The model under review builds one solid part; all positions refer to its coordinate system, in mm. Face numbers are marked on the shaded views. Give positions to 0.01 mm unless a question says otherwise; leave off trailing zeros. Order: outer loops, then holes, each group sorted by start corner. A loop starts at its lowest first (then second) coordinate and runs counter-clockwise, first axis right, second up. Notation, with made-up numbers: (75.5, -6.5) - (93.5, -6.5) arc R8 cw to (93.5, -0.5) - close; hole circle Ø11 at (30.25, 31.25). An arc over 180 degrees is marked (long way). Use CSV: the item, a comma, the result in double quotes.
```python
from build123d import *

# Parameters (mm, degrees)
BOSS_EXTRUDE1_DEPTH = 12.7
SKETCH2_R           = 3.175
CUT_EXTRUDE1_DEPTH  = 26.4
SKETCH3_OUTSIDE_W   = 105.562
SKETCH3_OUTSIDE_H   = 45.872
CUT_EXTRUDE4_DEPTH  = 25.4


with BuildPart() as part:
    # Sketch1 → Boss-Extrude1 (new body, symmetric)
    with BuildSketch(Plane.XY):
        with BuildLine():
            Line((-20, 0), (-42.545, 0))
            Line((-42.545, 0), (-42.545, -25.4))
            Line((-42.545, -25.4), (42.545, -25.4))
            Line((42.545, -25.4), (42.545, 0))
            Line((42.545, 0), (20, 0))
            ThreePointArc((20, 0), (0, -20), (-20, 0))
        make_face()
    extrude(amount=BOSS_EXTRUDE1_DEPTH, both=True)

    # Sketch2 → Cut-Extrude1 (cut, through all)
    with BuildSketch(Plane(origin=(0, 0, 0), x_dir=(1, 0, 0), z_dir=(0, 1, 0))):
        with Locations((-31.2725, 0)):
            Circle(SKETCH2_R)
    cut_extrude1 = extrude(amount=-CUT_EXTRUDE1_DEPTH, mode=Mode.SUBTRACT)

    # Mirror1: Cut-Extrude1 across plane
    add(cut_extrude1.mirror(Plane(origin=(0, 0, 0), x_dir=(0, 0, 1), z_dir=(1, 0, 0))), mode=Mode.SUBTRACT)

    # Sketch3 outside → Cut-Extrude4 (cut)
    with BuildSketch(Plane.XZ.offset(25.4)):
        Rectangle(SKETCH3_OUTSIDE_W, SKETCH3_OUTSIDE_H)
        with BuildLine():
            Line((-29.845, 12.7), (29.845, 12.7))
            ThreePointArc((29.845, 12.7), (42.545, 0), (29.845, -12.7))
            Line((29.845, -12.7), (-29.845, -12.7))
            ThreePointArc((-29.845, -12.7), (-42.545, 0), (-29.845, 12.7))
        make_face(mode=Mode.SUBTRACT)
    extrude(amount=-CUT_EXTRUDE4_DEPTH, mode=Mode.SUBTRACT)


solid = part.part
```
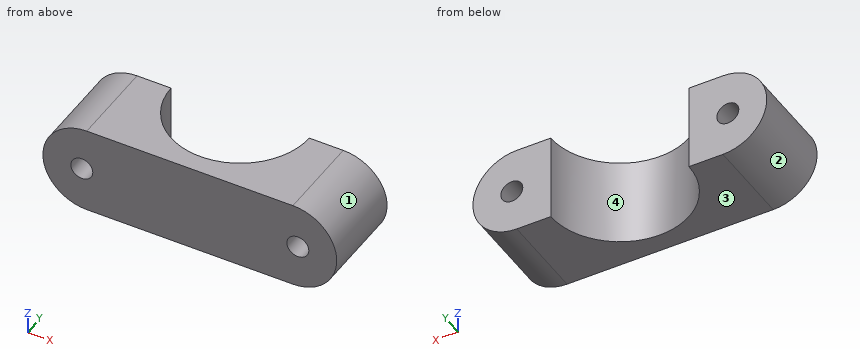
Item 1: Clearance check with flat-ended pins moving along their axes: pin 1 (1.5 mm diameter, centred on y = -8.5, z = 9.5, fed in from +X); pin 2 (5 mm diameter, centred on y = -21, z = -7, fed in from +X). State where each tip first meets the part, or that it passes through.
Results list:
pin 1,"stops at x = 39.05"
pin 2,"stops at x = 41.72"
Item 2: Mouldability with a two-part tool opening along X and no side actions: class the marked faces 1, 2, 3 and 4 as pulls with the +X half, pulls with the -X half, needs draft (parallel to the pull), parting line crosses it, or undercut.
Results list:
face 1,"pulls with the +X half"
face 2,"pulls with the -X half"
face 3,"needs draft"
face 4,"undercut"
Item 3: Take a section at A-A, the plane z = 0. Give the boundary of the cut face in (x, y) (1 decimal), and give its area (3 significant figures).
Results list:
outline,"(-42.5, -25.4) - (-34.4, -25.4) - (-34.4, 0) - (-42.5, 0) - close; (-28.1, -25.4) - (28.1, -25.4) - (28.1, 0) - (20, 0) arc R20 cw to (-20, 0) - (-28.1, 0) - close; (34.4, -25.4) - (42.5, -25.4) - (42.5, 0) - (34.4, 0) - close"
area,"1,210 mm2"
Item 4: Take a section at D-D, the plane x = 0. Give the boundary of the cut face in (y, z), and give its area (3 significant figures).
Results list:
outline,"(-25.4, -12.7) - (-20, -12.7) - (-20, 12.7) - (-25.4, 12.7) - close"
area,"137 mm2"
Item 5: Take a section at B-B, the plane y = -12.5. State how many separate pieces and enclosed holes the cut face has, and give its area (3 significant figures).
Results list:
separate pieces,"2"
enclosed holes,"2"
area,"1,170 mm2"
Item 6: Wall thickness on L1, parallel to X at y = -7.75, z = 0 (1 decimal); L2, parallel to X at y = -5.75, z = 0 (1 decimal); L3, parallel to X at y = -1.25, z = 3.5: over which ranges is each line inside the solid? List them lowest first.
Results list:
L1,"x = -42.5 to -34.4, -28.1 to -18.4, 18.4 to 28.1, 34.4 to 42.5"
L2,"x = -42.5 to -34.4, -28.1 to -19.2, 19.2 to 28.1, 34.4 to 42.5"
L3,"x = -42.05 to -19.96, 19.96 to 42.05"
